Work out the finished part from the listing and answer in its coordinate system (mm). Face numbers are marked on the shaded views. A direction names the side the tool comes from. Round coordinates to 2 decimals unless told otherwise and drop trailing zeros. Loops run counter-clockwise (first coordinate to the right, second up) from the corner with the lowest first, then second, coordinate; pieces in that order, holes last. Notation, with made-up numbers: (56.25, 43) -> (91.25, 43) arc R22 cw to (91.25, 68) -> close; hole circle Ø9 at (67, -23.5). An arc over 180 degrees is marked (long way). Use CSV: the item, a comma, the result in double quotes. Start each with the question number.
from build123d import *

# Parameters (mm, degrees)
PAD004_DEPTH    = 5.8
PAD007_DEPTH    = 3.5
SKETCH035_R     = 1.1
POCKET014_DEPTH = 2.5
FILLET001_R     = 1


with BuildPart() as part:
    # Sketch037 → Pad004 (new body, symmetric)
    with BuildSketch(Plane.YZ):
        Polygon((-16, 0), (-16, 1.6), (-11.75, 1.6), (-11.75, 5), (11.75, 5), (11.75, 1.6), (16, 1.6), (16, 0), (11.75, 0), (11.75, -15.3), (-6.25, -15.3), (-11.75, -13), (-11.75, 0), align=None)
    extrude(amount=PAD004_DEPTH, both=True)

    # Sketch006 (on DatumPlane) → Pad007 (join)
    with BuildSketch(Plane.XY.offset(5)):
        with BuildLine():
            Line((-3.35, -1.3266714218), (-3.35, -0.0999999323))
            ThreePointArc((3.35, -0.1000001307), (9.92e-08, 3.25), (-3.35, -0.0999999323))
            Line((3.35, -1.3266714218), (3.35, -0.1000001307))
            ThreePointArc((-3.35, -1.3266714218), (0, -11.75), (3.35, -1.3266714218))
        make_face()
    extrude(amount=PAD007_DEPTH)

    # Sketch035 → Pocket014 (cut, symmetric)
    with BuildSketch(Plane.XY):
        with Locations((0, 13.9)):
            Circle(SKETCH035_R)
        with Locations((0, -13.9)):
            Circle(SKETCH035_R)
    extrude(amount=POCKET014_DEPTH, both=True, mode=Mode.SUBTRACT)

    # Fillet001
    fillet001_edges = [part.edges().sort_by_distance(p)[0] for p in [
        (5.8, 16, 0.8),
        (-5.8, 16, 0.8),
        (5.8, -16, 0.8),
        (-5.8, -16, 0.8),
    ]]
    fillet(fillet001_edges, radius=FILLET001_R)


solid = part.part
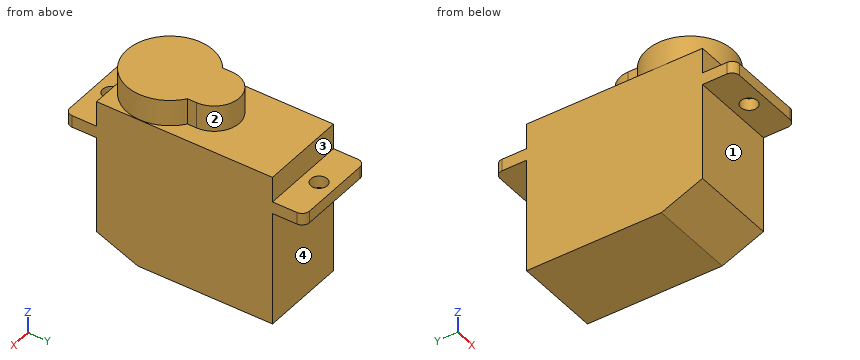
Q1. Section C-C, the plane z = 4 is taken. Write down the section's boundary in (x, y), and give its area (3 significant figures).
Q2. Which of the six approach directions +Z, -Z, +X, -X, +Y, -Y give full straight-line access (tool end or side, diameter ignored) to the marked faces 1, 2, 3 and 4?
Q3. Section D-D, the plane y = 7.5 is taken. Write down the section's boundary in (x, z), and give its area (3 significant figures).
Q4. Each of these flat-tipped pins is pushed along its axis until it touches: pin 1 (6 mm diameter, centred on x = 2, z = -5, fed in from -Y); pin 2 (2 mm diameter, centred on x = -2, y = 14, fed in from -Z); pin 3 (0.6 mm diameter, centred on y = -0.5, z = 7.5, fed in from +X). Where does it stop, or does it pass through?
Q5. Straight lines are drawn through the part: line 1 (Y direction, x = 0, z = 0.9); line 2 (X direction, y = 13.9, z = 0.95); line 3 (Z direction, x = -4.5, y = 1.5). For each, find the intervals that lie inside material, in ascending order. Write a range as from..to.
Q6. Section B-B, the plane x = 2.75 is taken. Write down the section's boundary in (y, z).
Q7. Section A-A, the plane y = -13.9 is taken. Write down the section's boundary in (x, z).
Report:
1,outline,"(-5.8, -11.75) -> (5.8, -11.75) -> (5.8, 11.75) -> (-5.8, 11.75) -> close"
1,area,"273 mm²"
2,face 1,"-Z, +X, -X, -Y"
2,face 2,"+Z, +Y"
2,face 3,"+Z, +X, -X, +Y"
2,face 4,"-Z, +X, -X, +Y"
3,outline,"(-5.8, -15.3) -> (5.8, -15.3) -> (5.8, 5) -> (-5.8, 5) -> close"
3,area,"235 mm²"
4,pin 1,"stops at y = -11.75"
4,pin 2,"stops at z = 0"
4,pin 3,"stops at x = 3.35"
5,line 1,"y = -16..-15, -12.8..12.8, 15..16"
5,line 2,"x = -5.8..-1.1, 1.1..5.8"
5,line 3,"z = -15.3..5"
6,outline,"(-16, 0) -> (-11.75, 0) -> (-11.75, -13) -> (-6.25, -15.3) -> (11.75, -15.3) -> (11.75, 0) -> (16, 0) -> (16, 1.6) -> (11.75, 1.6) -> (11.75, 5) -> (1.81, 5) -> (1.81, 8.5) -> (-11.05, 8.5) -> (-11.05, 5) -> (-11.75, 5) -> (-11.75, 1.6) -> (-16, 1.6) -> close"
7,outline,"(-5.8, 0) -> (-1.1, 0) -> (-1.1, 1.6) -> (-5.8, 1.6) -> close; (1.1, 0) -> (5.8, 0) -> (5.8, 1.6) -> (1.1, 1.6) -> close"
